The drawing under review shows one solid part. Ordinate dimensions are in mm from its lowest x, y, z. A direction names the side the tool comes from. Round coordinates to 2 decimals unless told otherwise and drop trailing zeros. Write each loop counter-clockwise with the first axis right and the second up, starting at its lowest first coordinate (ties: lowest second). Pieces come first, ordered by that corner, then holes. Notation, with made-up numbers: (26, 62.25) -> (44, 62.25) arc R29 ccw to (44, 84.25) -> close; hole circle Ø1 at (11.25, 21.25). An arc over 180 degrees is marked (long way). Use CSV: the item, a comma, the result in double quotes. Start each with the question number.
1) Take a section at B-B, the plane z = 2.4. Give the boundary of the cut face in (x, y), then the cut area to 3 significant figures.
2) Machinability: for the marked faces 1 and 2, which of the approach directions +Z, -Z, +X, -X, +Y, -Y give a long, thin tool a straight path to every point of the face, cutting with its end or side? Answer none if there is none.
3) For pin 1 Ø0.6 at (x, y) = (2.5, 0) entering from -Z; pin 2 Ø0.6 at (x, y) = (2.5, 0) entering from +Z; pin 3 Ø0.6 at (y, z) = (0, 1) entering from -X, all flat-tipped, find the tip position at first contact; note any pin that passes through.
4) Take a section at C-C, the plane y = 5.75. Give the boundary of the cut face in (x, z).
5) Take a section at D-D, the plane y = 1.25. Give the boundary of the cut face in (x, z).
6) Take a section at A-A, the plane x = 2.4. Give the boundary of the cut face in (y, z), then the cut area to 3 significant figures.
7) Wall thickness on probe 1 along Y at (x, z) = (2.1, 3.1); probe 2 along Y at (x, z) = (0.55, 2.3); probe 3 along X at (y, z) = (2.75, 3.05): over which ranges is each line inside the solid? List them lowest first. Write a range as [from, to].
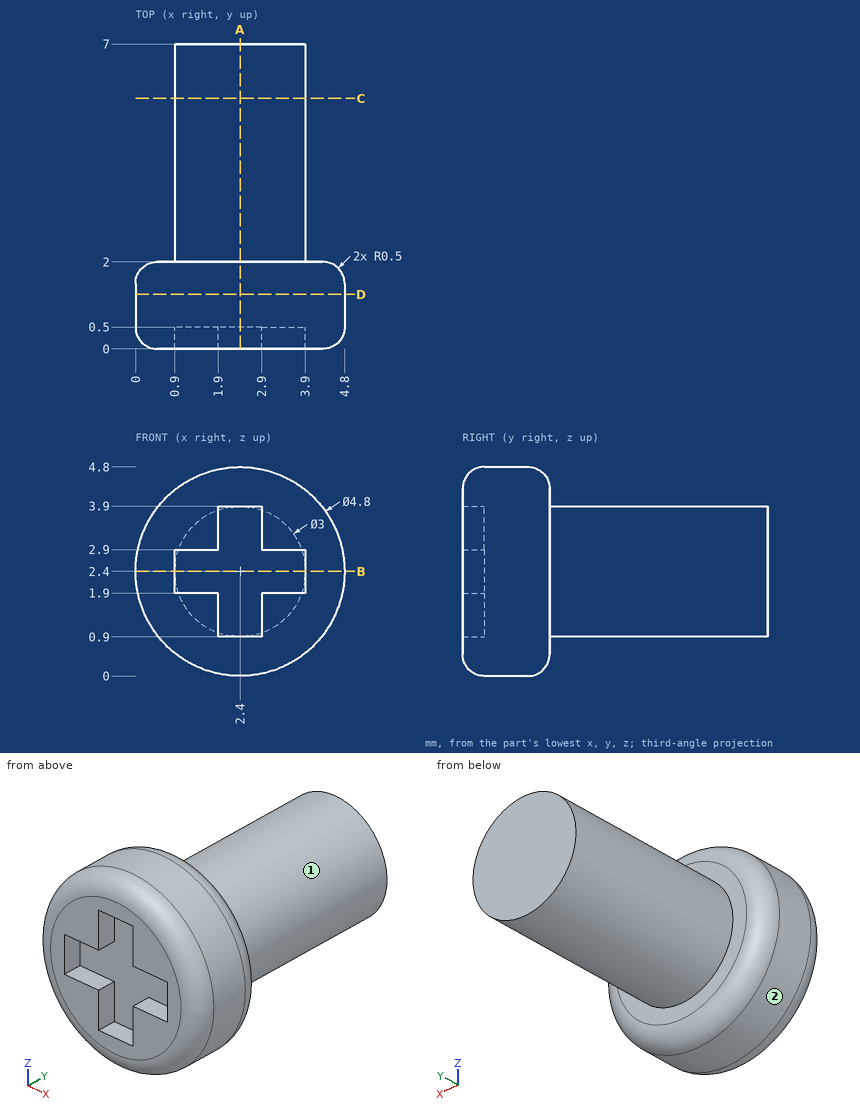
Values found:
1,outline,"(0, 0.5) arc R0.5 ccw to (0.5, 0) -> (0.9, 0) -> (0.9, 0.5) -> (3.9, 0.5) -> (3.9, 0) -> (4.3, 0) arc R0.5 ccw to (4.8, 0.5) -> (4.8, 1.5) arc R0.5 ccw to (4.3, 2) -> (3.9, 2) -> (3.9, 7) -> (0.9, 7) -> (0.9, 2) -> (0.5, 2) arc R0.5 ccw to (0, 1.5) -> close"
1,area,"22.9 mm²"
2,face 1,"+Y"
2,face 2,"+Y, -Y"
3,pin 1,"z = 0.04"
3,pin 2,"z = 4.76"
3,pin 3,"x = 0.42"
4,outline,"circle Ø3 at (2.4, 2.4)"
5,outline,"circle Ø4.8 at (2.4, 2.4)"
6,outline,"(0, 0.5) arc R0.5 ccw to (0.5, 0) -> (1.5, 0) arc R0.5 ccw to (2, 0.5) -> (2, 0.9) -> (7, 0.9) -> (7, 3.9) -> (2, 3.9) -> (2, 4.3) arc R0.5 ccw to (1.5, 4.8) -> (0.5, 4.8) arc R0.5 ccw to (0, 4.3) -> (0, 3.9) -> (0.5, 3.9) -> (0.5, 0.9) -> (0, 0.9) -> close"
6,area,"22.9 mm²"
7,probe 1,"[0.5, 7]"
7,probe 2,"[0, 2]"
7,probe 3,"[1.05, 3.75]"
